CAD build for the part. Positions are in the model's coordinates, mm. A direction names the side the tool comes from. Coordinates: 2 decimals unless noted, no trailing zeros. Order: outer loops, then holes, each group sorted by start corner. A loop starts at its lowest first (then second) coordinate and runs counter-clockwise, first axis right, second up. Notation, with made-up numbers: M 51.5,10.25 L 55.5,10.25 A29 ccw 55.5,34.25 Z; hole C 86,-22 d10. An arc over 180 degrees is marked long. Write item = value, one per line. Start each with the question number.
Autodesk Inventor part; units mm, degrees
ref_plane "YZ Plane" through (0, 0, 0) normal (1, 0, 0) x (0, 1, 0)
ref_plane "XZ Plane" through (0, 0, 0) normal (0, 1, 0) x (-1, 0, 0)
ref_plane "XY Plane" through (0, 0, 0) normal (0, 0, 1) x (1, 0, 0)
sketch "Sketch1" plane through (0, 0, 0) normal (0, 0, 1) x (1, 0, 0)
  line L0 (0, 0) -> (50, 0)
  line L1 (50, 0) -> (50, 80) construction
  line L2 (50, 80) -> (0, 80)
  line L3 (0, 80) -> (0, 0)
  circle A0 centre (50, 40) radius 40 construction
  arc A1 (50, 0) -> (50, 80) centre (50, 40) ccw
  dimension "d0" = 50
  dimension "d1" = 80
  dimension "d2" = 80
extrude "Extrusion1" add sketch "Sketch1" along normal blind 40
sketch "Sketch2" plane through (0, 0, 0) normal (0, 0, -1) x (-1, 0, 0)
  line L0 (-50, 80) -> (0, 80)
  arc A0 (-50, 80) -> (-50, 0) centre (-50, 40) ccw
  line L1 (0, 0) -> (-50, 0)
  line L2 (0, 75) -> (-50, 75)
  arc A1 (-50, 75) -> (-50, 5) centre (-50, 40) ccw
  line L3 (-50, 5) -> (0, 5)
  line L4 (0, 75) -> (0, 5)
  line L5 (0, 80) -> (0, 0)
  dimension "d5" = 5
extrude "Extrusion2" cut sketch "Sketch2" against normal blind 35 contours L4 L3 A1 L2
sketch "Sketch3" plane through (0, 0, 40) normal (-1, 0, 0) x (0, 0, 1)
  line L0 (0, 80) -> (0, 0)
  line L1 (-40, 5) -> (-40, 75)
  line L2 (0, 80) -> (-40, 80)
  line L3 (-40, 80) -> (-40, 70)
  line L4 (-40, 70) -> (0, 70)
  line L5 (0, 70) -> (0, 80)
  line L6 (0, 80) -> (-10, 80)
  line L7 (-10, 80) -> (-10, 50)
  line L8 (-10, 50) -> (0, 50)
  line L9 (0, 50) -> (0, 80)
  line L10 (-40, 0) -> (0, 0)
  dimension "d8" = 10
  dimension "d9" = 10
  dimension "d10" = 50
extrude "Extrusion3" add sketch "Sketch3" against normal blind 5
sketch "Sketch4" plane through (0, 0, 0) normal (0, 0, -1) x (-1, 0, 0)
  arc A0 (-50, 80) -> (-50, 0) centre (-50, 40) ccw
  line L0 (-50, 80) -> (0, 80)
  arc A1 (-50, 80) -> (-50, 0) centre (-50, 40) ccw
  line L1 (-50, 0) -> (-50, 80)
  line L2 (-50, 40) -> (-40, 80)
  line L3 (-50, 80) -> (0, 80)
  line L4 (-40, 80) -> (-50, 80)
  line L5 (-50, 40) -> (-40, 0)
  line L6 (0, 0) -> (-50, 0)
  line L7 (-40, 0) -> (-50, 0)
  dimension "d15" = 10
extrude "Extrusion4" cut sketch "Sketch4" against normal blind 10
sketch "Sketch8" plane through (0, 0, 35) normal (0, 0, -1) x (-1, 0, 0)
  circle A0 centre (-50, 40) radius 4.5
  circle A1 centre (-50, 40) radius 15
  line L0 (0, 0) -> (-40, 0)
  line L1 (0, 50) -> (0, 5)
  dimension "d25" = 30
  dimension "d34" = 40
  dimension "d35" = 50
  dimension "d36" = 9
extrude "Extrusion8" add sketch "Sketch8" along normal blind 5
sketch "Sketch9" plane through (0, 0, 35) normal (0, 0, -1) x (-1, 0, 0)
  line L0 (0, 80) -> (0, 0)
  circle A0 centre (-11.5, 30) radius 4.5
  line L1 (0, 0) -> (-40, 0)
  circle A1 centre (-11.5, 30) radius 10
  dimension "d28" = 9
  dimension "d29" = 30
  dimension "d30" = 11.5
  dimension "d33" = 20
extrude "Extrusion9" add sketch "Sketch9" along normal blind 5
sketch "Sketch11" plane through (0, 0, 35) normal (0, 0, -1) x (-1, 0, 0)
  circle A0 centre (-15, 65) radius 10
  circle A1 centre (-15, 65) radius 2.5
  line L0 (-41.25, 75) -> (-5, 75)
  line L1 (-5, 50) -> (-5, 70)
  point P0 (0, 0)
  dimension "d39" = 20
  dimension "d40" = 5
extrude "Extrusion10" add sketch "Sketch11" along normal blind 35
sketch "Sketch13" plane through (0, 0, 40) normal (0, 0, 1) x (1, 0, 0)
  circle A0 centre (50, 40) radius 15
  circle A1 centre (11.5, 30) radius 10
  circle A2 centre (11.5, 30) radius 4.5
  circle A3 centre (11.5, 30) radius 2.5
  circle A4 centre (50, 40) radius 4.5
  circle A5 centre (50, 40) radius 2.5
  point P0 (0, 0)
  dimension "d46" = 5
  dimension "d47" = 5
extrude "Extrusion12" cut sketch "Sketch13" against normal through all contours A3 | A5
properties part number "FA005" material "ABS Plastic"
1. Mould opens along Y. For faces 1 (the flat face through (44, 41, 40)), 2 (the flat face through (25, 0, 20)), 3 (the cylindrical face through (52.31, 39.04, 37.53)), 4 (the flat face through (2, 70, 15)) say: released by +Y, released by -Y, zero draft, split by the parting line, or undercut.
2. Flat gauge pins, fed straight in: pin 1 (4 mm diameter, centred on x = 3, y = 60.5, fed in from -Z); pin 2 (10 mm diameter, centred on y = 60.5, z = 27, fed in from +X); pin 3 (8 mm diameter, centred on x = 11.5, y = 30, fed in from -Z). Where does each tip first touch, or does it go through?
3. Slice it at C-C (x = 28). Write the cut outline in (y, z).
4. Probe L1, parallel to Y at x = 18, z = 5.5; L2, parallel to Y at x = 11, z = 31; L3, parallel to Y at x = 50, z = 38.65. List the from-to ranges inside material, lowest first.
5. Slice it at D-D (y = 17). Write the cut outline in (x, z), plus the area to 3 significant figures.
6. 3-axis set-ups, long thin cutter, end or side, ignore diameter. For faces 5 (the flat face through (15, 65, 35)), 6 (the flat face through (40.634, 2.535, 4.93)), 7 (the flat face through (25, 80, 20)), 8 (the flat face through (7, 28, 30)): which of +Z, -Z, +X, -X, +Y, -Y reach the whole face in a straight line?
Calculated:
q1.face_1 = zero draft
q1.face_2 = released by -Y
q1.face_3 = undercut
q1.face_4 = undercut
q2.pin_1 = 30
q2.pin_2 = 86.87
q2.pin_3 = 35
q3.outline = M 0,0 L 5,0 L 5,35 L 75,35 L 75,0 L 80,0 L 80,40 L 0,40 Z
q4.L1 = 0 to 5, 55.46 to 74.54, 75 to 80
q4.L2 = 0 to 5, 20.01 to 25.53, 34.47 to 39.99, 55.83 to 74.17, 75 to 80
q4.L3 = 0 to 37.5, 42.5 to 80
q5.outline = M 0,35 L 76.38,35 L 76.38,10 L 82.73,10 L 82.73,40 L 0,40 Z
q5.area = 572 mm²
q6.face_5 = -Z
q6.face_6 = -Z, +X, -Y
q6.face_7 = +Z, -Z, +X, -X, +Y
q6.face_8 = -Z, -X
